Verification items for the finished model (mm, model axes). Coordinates: 2 decimals unless noted, no trailing zeros. Write each loop counter-clockwise with the first axis right and the second up, starting at its lowest first coordinate (ties: lowest second). Pieces come first, ordered by that corner, then holes. Notation, with made-up numbers: (51, -32) - (89, -32) arc R12 ccw to (89, -11) - close; hole circle Ø6 at (80.5, 48.5). An arc over 180 degrees is marked (long way). Answer as CSV lines item,"result". Start each with the question number.
```python
from build123d import *

# Parameters (mm, degrees)
EXTRUSION1_DEPTH           = 60
EXTRUSION2_START           = -10
ESQUISSE2_W                = 7.046962448
ESQUISSE2_H                = 15
EXTRUSION2_DEPTH           = 73.139279043
R_P_TITION_LIN_AIRE1_COUNT = 2
R_P_TITION_LIN_AIRE1_PITCH = 30
ESQUISSE3_R                = 1.5
EXTRUSION3_DEPTH           = 63.139279043
R_P_TITION_LIN_AIRE2_COUNT = 3
R_P_TITION_LIN_AIRE2_PITCH = 20


with BuildPart() as part:
    # Esquisse1 → Extrusion1 (new body)
    with BuildSketch(Plane.XY):
        with BuildLine():
            Line((0, 0), (16, 0))
            Line((16, 0), (16, 0.7))
            Line((16, 0.7), (1.268857754, 0.7))
            ThreePointArc((1.268857754, 0.7), (-0.724568837, 2.813392554), (0, 0))
        make_face()
    extrude(amount=EXTRUSION1_DEPTH)

    # Esquisse2 → Extrusion2 (cut, through all)
    with BuildSketch(Plane(origin=(0, 0.7, 0), x_dir=(1, 0, 0), z_dir=(0, 1, 0)).offset(EXTRUSION2_START)):
        with Locations((-1.523481224, -52.5)):
            Rectangle(ESQUISSE2_W, ESQUISSE2_H)
    extrusion2 = extrude(amount=EXTRUSION2_DEPTH, mode=Mode.SUBTRACT)

    # Répétition linéaire1: Extrusion2 ×2
    with Locations(*[(0, 0, -i * R_P_TITION_LIN_AIRE1_PITCH) for i in range(1, R_P_TITION_LIN_AIRE1_COUNT)]):
        add(extrusion2, mode=Mode.SUBTRACT)

    # Esquisse3 → Extrusion3 (cut, through all)
    with BuildSketch(Plane(origin=(0, 0.7, 0), x_dir=(1, 0, 0), z_dir=(0, 1, 0))):
        with Locations(Location((11, -50, 0), (0, 0, 180))):
            Circle(ESQUISSE3_R)
    extrusion3 = extrude(amount=-EXTRUSION3_DEPTH, mode=Mode.SUBTRACT)

    # Répétition linéaire2: Extrusion3 ×3
    with Locations(*[(0, 0, -i * R_P_TITION_LIN_AIRE2_PITCH) for i in range(1, R_P_TITION_LIN_AIRE2_COUNT)]):
        add(extrusion3, mode=Mode.SUBTRACT)


solid = part.part
```
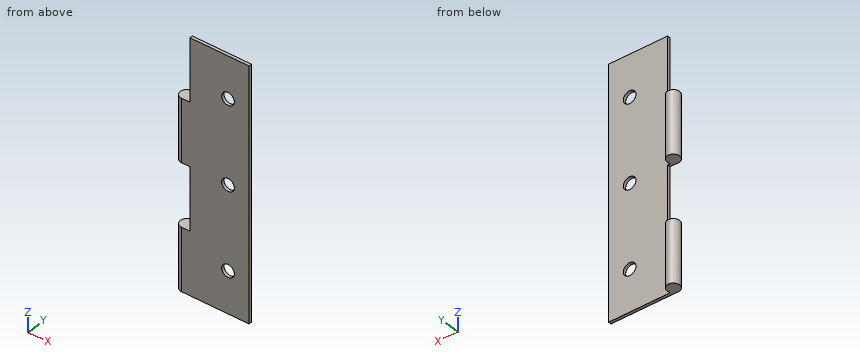
1. Scan lines: line 1 along Z through (x, y) = (11, 0.55); line 2 along Z through (x, y) = (0, 0.6); line 3 along Y through (x, z) = (9.75, 54.5). Record each from-to range of solid material in increasing order. Write a range as from..to.
2. Cross-section at B-B (z = 50). Record the cut outline in (x, y).
3. Depth check by flat-ended pin: P1, Ø6, axis at x = 7, z = 52, coming from the +Y side; P2, Ø1.5, axis at x = 1, y = 1, coming from the +Z side. Enter the tip coordinate at first touch or a pass-through.
4. Cross-section at A-A (x = 11). Record the cut outline in (y, z).
5. Cross-section at C-C (y = 1.5). Record the cut outline in (x, z), and give its area (3 significant figures).
6. Cross-section at D-D (x = 14.75). Record the cut outline in (y, z), and give its area (3 significant figures).
Completed:
1,line 1,"z = 0..8.5, 11.5..28.5, 31.5..48.5, 51.5..60"
1,line 2,"z = 0..15, 30..45"
1,line 3,"y = 0..0.7"
2,outline,"(2, 0) - (9.5, 0) - (9.5, 0.7) - (2, 0.7) - close; (12.5, 0) - (16, 0) - (16, 0.7) - (12.5, 0.7) - close"
3,P1,"stops at y = 0.7"
3,P2,"stops at z = 45"
4,outline,"(0, 0) - (0.7, 0) - (0.7, 8.5) - (0, 8.5) - close; (0, 11.5) - (0.7, 11.5) - (0.7, 28.5) - (0, 28.5) - close; (0, 31.5) - (0.7, 31.5) - (0.7, 48.5) - (0, 48.5) - close; (0, 51.5) - (0.7, 51.5) - (0.7, 60) - (0, 60) - close"
5,outline,"(-1.5, 0) - (1.5, 0) - (1.5, 15) - (-1.5, 15) - close; (-1.5, 30) - (1.5, 30) - (1.5, 45) - (-1.5, 45) - close"
5,area,"90.0 mm2"
6,outline,"(0, 0) - (0.7, 0) - (0.7, 60) - (0, 60) - close"
6,area,"42.0 mm2"
